Design review of the part built by this model. Coordinates are the model's own, in mm. Face numbers are marked on the shaded views. A direction names the side the tool comes from. Coordinates: 2 decimals unless noted, no trailing zeros. Loops run counter-clockwise (first coordinate to the right, second up) from the corner with the lowest first, then second, coordinate; pieces in that order, holes last. Notation, with made-up numbers: (39, 41.25) - (82, 41.25) arc R20 ccw to (82, 63.25) - close; hole circle Ø10 at (-19, 38.5). An arc over 180 degrees is marked (long way). Answer in a Markdown table with one row per item. Add a question column.
(1) We need section A-A, the plane x = 4.75. Write out the cut boundary in (y, z).
(2) Clearance check with flat-ended pins moving along their axes: pin 1 (1.5 mm diameter, centred on x = 7.5, y = 1.5, fed in from -Z); pin 2 (1.5 mm diameter, centred on x = 8.5, z = 0.5, fed in from +Y); pin 3 (1.5 mm diameter, centred on x = 8, z = -0.5, fed in from -Y). State where each tip first meets the part, or that it passes through.
(3) We need section B-B, the plane z = -3. Write out the cut boundary in (x, y).
(4) We need section C-C, the plane y = 2. Write out the cut boundary in (x, z).
(5) We need section D-D, the plane z = 0. Write out the cut boundary in (x, y).
(6) For the marked faces 1, 2 and 3, list the 3-axis set-ups (+Z, -Z, +X, -X, +Y, -Y) from which the entire face can be reached by the end or side of a thin tool; tool diameter is ignored.
(7) The part is to be moulded in two halves that separate along X. For the marked faces 4, 5 and 6, say which applies: released by +X, released by -X, zero draft, split by the parting line, or undercut.
(8) To check wall thickness, follow L1, parallel to Z at x = 4.75, y = 1; L2, parallel to X at y = 1.3, z = 2.5; L3, parallel to Y at x = -0.5, z = -0.75. State the ranges of each line that lie inside material, in increasing order. Write a range as [from, to].
Autodesk Inventor part; units mm, degrees
ref_plane "YZ Plane" through (0, 0, 0) normal (1, 0, 0) x (0, 1, 0)
ref_plane "XZ Plane" through (0, 0, 0) normal (0, 1, 0) x (-1, 0, 0)
ref_plane "XY Plane" through (0, 0, 0) normal (0, 0, 1) x (1, 0, 0)
sketch "Sketch1" plane through (0, 0, 0) normal (0, 1, 0) x (-1, 0, 0)
  circle A0 centre (0, 0) radius 4
  line L0 (0, 4) -> (-6.5, 4)
  line L1 (-6.5, 4) -> (-6.5, -4)
  line L2 (-6.5, -4) -> (0, -4)
  line L3 (0, -4) -> (0, 4)
  circle A1 centre (-4.75, 2.75) radius 1.1
  circle A2 centre (-4.75, -2.75) radius 1.1
  point P0 (-6.5, 0)
  dimension "d0" = 8
  dimension "d1" = 6.5
  dimension "d2" = 5.5
  dimension "d3" = 2.75
  dimension "d4" = 1.75
  dimension "d5" = 1.75
  dimension "d6" = 2.2
  dimension "d7" = 2.2
extrude "Extrusion1" add sketch "Sketch1" along normal blind 4
sketch "Sketch2" plane through (6.5, 0, 4) normal (1, 0, 0) x (0, 0, -1)
  line L0 (2.5, 3.5) -> (5.5, 3.5)
  line L1 (5.5, 3.5) -> (5.5, 0.5)
  line L2 (5.5, 0.5) -> (2.5, 0.5)
  line L3 (2.5, 0.5) -> (2.5, 3.5)
  line L4 (0, 4) -> (8, 4)
  line L5 (8, 0) -> (8, 4)
  point P0 (4, 0)
  dimension "d10" = 3
  dimension "d11" = 3
  dimension "d12" = 0.5
  dimension "d13" = 5.5
extrude "Extrusion2" add sketch "Sketch2" along normal blind 4
sketch "Sketch3" plane through (0, 4, 0) normal (0, 1, 0) x (1, 0, 0)
  circle A0 centre (0, 0) radius 2.05
  dimension "d16" = 4.1
extrude "Extrusion3" cut sketch "Sketch3" against normal blind 0.1
sketch "Sketch4" plane through (10.5, 0, 4) normal (1, 0, 0) x (0, 0, -1)
  circle A0 centre (4, 2) radius 1.1
  point P0 (4, 0)
  dimension "d19" = 2.2
extrude "Extrusion4" add sketch "Sketch4" along normal blind 10
equation "\"d5\" = d4"
equation "\"d6\" = d7"
properties part number "CapacitiveSensor"
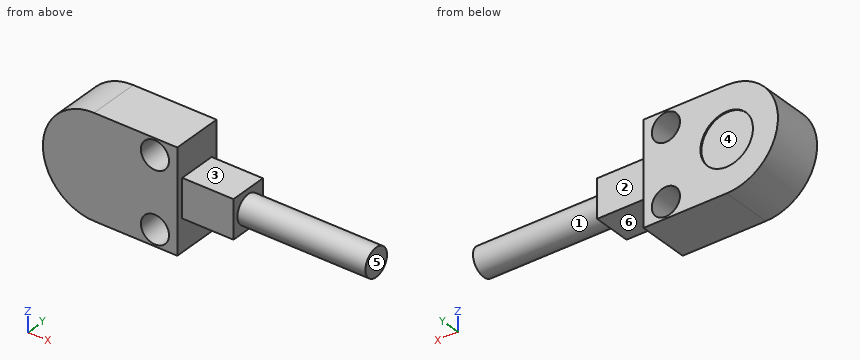
Responses:
| question | item | result |
|---|---|---|
| 1 | outline | (0, -4) - (4, -4) - (4, -3.85) - (0, -3.85) - close; (0, -1.65) - (4, -1.65) - (4, 1.65) - (0, 1.65) - close; (0, 3.85) - (4, 3.85) - (4, 4) - (0, 4) - close |
| 2 | pin 1 | stops at z = -1.5 |
| 2 | pin 2 | stops at y = 3.5 |
| 2 | pin 3 | stops at y = 0.5 |
| 3 | outline | (-2.65, 0) - (3.68, 0) - (3.68, 4) - (-2.65, 4) - close; (5.82, 0) - (6.5, 0) - (6.5, 4) - (5.82, 4) - close |
| 4 | outline | (0, -4) - (6.5, -4) - (6.5, -1.5) - (10.5, -1.5) - (10.5, -1.1) - (20.5, -1.1) - (20.5, 1.1) - (10.5, 1.1) - (10.5, 1.5) - (6.5, 1.5) - (6.5, 4) - (0, 4) arc R4 ccw to start; hole circle Ø2.2 at (4.75, -2.75); hole circle Ø2.2 at (4.75, 2.75) |
| 5 | outline | (-4, 0) - (6.5, 0) - (6.5, 0.5) - (10.5, 0.5) - (10.5, 0.9) - (20.5, 0.9) - (20.5, 3.1) - (10.5, 3.1) - (10.5, 3.5) - (6.5, 3.5) - (6.5, 4) - (2.05, 4) - (2.05, 3.9) - (-2.05, 3.9) - (-2.05, 4) - (-4, 4) - close |
| 6 | face 1 | +X |
| 6 | face 2 | +Z, -Z, +X, +Y |
| 6 | face 3 | +Z, +X, +Y, -Y |
| 7 | face 4 | undercut |
| 7 | face 5 | released by +X |
| 7 | face 6 | zero draft |
| 8 | L1 | z = [-4, -3.85], [-1.65, 1.65], [3.85, 4] |
| 8 | L2 | x = [-3.12, 3.68], [5.82, 6.5] |
| 8 | L3 | y = [0, 3.9] |
